Verification items for the finished model (mm, model axes). Face numbers are marked on the shaded views. A direction names the side the tool comes from. Round coordinates to 2 decimals unless told otherwise and drop trailing zeros. Order: outer loops, then holes, each group sorted by start corner. A loop starts at its lowest first (then second) coordinate and runs counter-clockwise, first axis right, second up. Notation, with made-up numbers: (87, 2.5) -> (135, 2.5) arc R23 ccw to (135, 30.5) -> close; hole circle Ø1 at (4, 40). An arc over 180 degrees is marked (long way). Return JSON: item names as keys, results as strings. Group by question number.
1) Depth check by flat-ended pin: pin 1 (8 mm diameter, centred on y = 4.5, z = 0, fed in from +X); pin 2 (4 mm diameter, centred on y = 4, z = -0.5, fed in from -X); pin 3 (2 mm diameter, centred on x = 7.5, y = 7, fed in from -Z); pin 4 (8 mm diameter, centred on y = 14.5, z = 5, fed in from +X). Enter the tip coordinate at first touch or a pass-through.
2) Section check B-B on y = 13.25. Enter the section's corners in (x, z).
3) Section check A-A on y = 18. Enter the section's corners in (x, z).
4) Scan lines: L1, parallel to X at y = 19.6, z = 0; L2, parallel to Y at x = -9, z = -5.25. Record each from-to range of solid material in increasing order.
5) Draft check along X on the marked faces 1, 2 and 3. Enter one of: pulls with the +X half, pulls with the -X half, needs draft (parallel to the pull), parting line crosses it, or undercut.
6) Tool access check on the marked faces 4 and 5. Record the directions out of +Z, -Z, +X, -X, +Y, -Y that give a thin tool (end or side, any length) a straight path to the whole face; none if there is none.
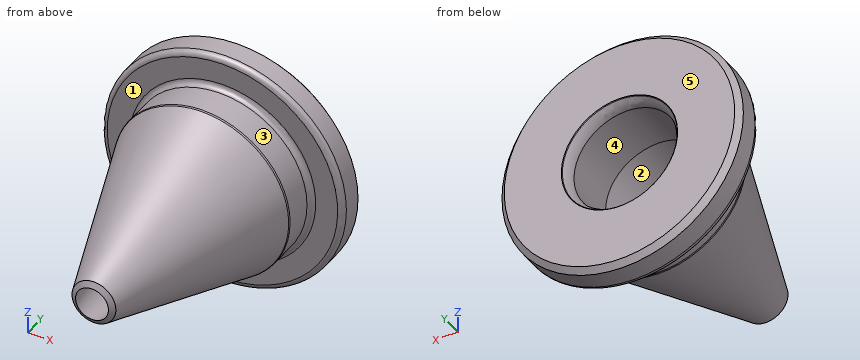
```python
from build123d import *

# Parameters (mm, degrees)
FL_CHE_VERSCHIEBEN1_BY          = 1
AUFSATZ_LINEAR_START            = -2.8
SKIZZE2_R                       = 11
SKIZZE2_R_2                     = 4.8
AUFSATZ_LINEAR_AUSTRAGEN1_DEPTH = 2.8
VERRUNDUNG1_R                   = 0.5
FASE1_SIZE                      = 0.5
VERRUNDUNG2_R                   = 1.5


with BuildPart() as part:
    # Skizze1 → Rotation1 (revolve)
    with BuildSketch(Plane.XY, mode=Mode.PRIVATE) as rotation1_sk:
        Polygon((1.5, 0), (4.8, 17), (4.8, 22), (8, 22), (8, 17), (2, 0.3), align=None)
    revolve(rotation1_sk.sketch.rotate(Axis((0, 0, 0), (0, 1, 0)), 270), axis=Axis((0, 0, 0), (0, 1, 0)))

    # Fläche verschieben1: a face moved outward by 1.0
    extrude(part.faces().sort_by_distance((-6.4, 22, 0))[0], amount=FL_CHE_VERSCHIEBEN1_BY, dir=(0, 1, 0))

    # Skizze2 → Aufsatz-Linear austragen1 (add)
    with BuildSketch(Plane(origin=(0, 23, 0), x_dir=(1, 0, 0), z_dir=(0, 1, 0)).offset(AUFSATZ_LINEAR_START)):
        with Locations(Location((0, 0, 0), (0, 0, 270))):
            Circle(SKIZZE2_R)
        with Locations(Location((0, 0, 0), (0, 0, 270))):
            Circle(SKIZZE2_R_2, mode=Mode.SUBTRACT)
    extrude(amount=AUFSATZ_LINEAR_AUSTRAGEN1_DEPTH)

    # Verrundung1
    verrundung1_edges = [part.edges().sort_by_distance(p)[0] for p in [
        (0, 20.2, -8),
        (0, 20.2, -11),
        (0, 17, -8),
    ]]
    fillet(verrundung1_edges, radius=VERRUNDUNG1_R)

    # Fase1
    fase1_edges = [part.edges().sort_by_distance(p)[0] for p in [
        (0, 23, -11),
        (0, 23, -4.8),
    ]]
    chamfer(fase1_edges, length=FASE1_SIZE)

    # Verrundung2
    verrundung2_edges = [part.edges().sort_by_distance(p)[0] for p in [
        (0, 22.5, -4.8),
    ]]
    fillet(verrundung2_edges, radius=VERRUNDUNG2_R)


solid = part.part
```
Check result:
{
 "1": {"pin 1": "x = 4.95", "pin 2": "x = -4.03", "pin 3": "through", "pin 4": "x = 7.77"},
 "2": {"outline": "circle Ø13.31 at (0, 0); hole circle Ø8.14 at (0, 0)"},
 "3": {"outline": "circle Ø16 at (0, 0); hole circle Ø9.6 at (0, 0)"},
 "4": {"L1": "-8 to -4.8, 4.8 to 8", "L2": "20.2 to 23"},
 "5": {"face 1": "needs draft", "face 2": "undercut", "face 3": "parting line crosses it"},
 "6": {"face 4": "+Y", "face 5": "+Z, -Z, +X, -X, +Y"}
}
